Geometry: final body of the model. Coordinates: model frame, mm. Round coordinates to 2 decimals unless told otherwise and drop trailing zeros. Write each loop counter-clockwise with the first axis right and the second up, starting at its lowest first coordinate (ties: lowest second). Pieces come first, ordered by that corner, then holes. Notation, with made-up numbers: M -37.75,23.25 L -10.75,23.25 A30 cw -10.75,62.25 Z; hole C 17,33 d7. An arc over 180 degrees is marked long. Answer as CSV lines item,"result". Start each with the question number.
Q1. Mould query, pull axis Y, two halves, no side actions, for faces 1 (the flat face through (-26.69, -18.86, 8.52)), 2 (the cylindrical face through (30.24, -3.65, -0.14)), 3 (the flat face through (26.69, 18.86, 8.52)). Classes: pulls with the +Y half, pulls with the -Y half, needs draft (parallel to the pull), parting line crosses it, or undercut.
Q2. Ray query, probe 1 along X at (y, z) = (-9, 3.5); probe 2 along Y at (x, z) = (17.5, 9.25); probe 3 along Y at (x, z) = (-29.5, 1.75). Return the intervals inside material, ascending.
Q3. Section query D-D on x = 35. Output: boundary loops of the cut face in (y, z), and give its area (3 significant figures).
Q4. Section query C-C on x = 0. Output: boundary loops of the cut face in (y, z).
Q5. Section query B-B on y = 0. Output: boundary loops of the cut face in (x, z), and give its area (3 significant figures).
Q6. First-contact query: pin 1 (10 mm diameter, centred on x = -28, z = 3, fed in from +Y); pin 2 (10 mm diameter, centred on x = -36, z = -6.5, fed in from -Y); pin 3 (8 mm diameter, centred on y = -21.5, z = 6, fed in from -X). Flat tips, straight axial feed; report the tip coordinate or a pass-through.
Q7. Section query A-A on z = -1.25. Output: boundary loops of the cut face in (x, y).
```python
from build123d import *

# Parameters (mm, degrees)
F0_R     = 6
F0_R_2   = 21
F1_DEPTH = 10
F2_SIZE  = 3


with BuildPart() as f1:
    # F0 (on Top) → F1 (new body)
    with BuildSketch(Plane.XY):
        with BuildLine():
            Line((41.428571, 13.552619), (12.857143, 27.105237))
            ThreePointArc((12.857143, 27.105237), (0, 30), (-12.857143, 27.105237))
            Line((-12.857143, 27.105237), (-41.428571, 13.552619))
            ThreePointArc((-41.428571, 13.552619), (-50, 0), (-41.428571, -13.552619))
            Line((-41.428571, -13.552619), (-12.857143, -27.105237))
            ThreePointArc((-12.857143, -27.105237), (0, -30), (12.857143, -27.105237))
            Line((12.857143, -27.105237), (41.428571, -13.552619))
            ThreePointArc((41.428571, -13.552619), (50, 0), (41.428571, 13.552619))
        make_face()
        with Locations((-35, 0)):
            Circle(F0_R, mode=Mode.SUBTRACT)
        Circle(F0_R_2, mode=Mode.SUBTRACT)
        with Locations((35, 0)):
            Circle(F0_R, mode=Mode.SUBTRACT)
    extrude(amount=F1_DEPTH)

    # F2
    f2_edges = [f1.edges().sort_by_distance(p)[0] for p in [
        (-27.142857, -20.328928, 10),
        (0, -30, 10),
        (27.142857, -20.328928, 10),
    ]]
    chamfer(f2_edges, length=F2_SIZE)

    # F3: F1 across face


with BuildPart() as f1_1:
    add(f1.part)
    add(f1.part.mirror(Plane(origin=(0, 0, 0), x_dir=(1, 0, 0), z_dir=(0, 0, -1))))


solid = f1_1.part
```
Entries:
1,face 1,"pulls with the -Y half"
1,face 2,"undercut"
1,face 3,"pulls with the +Y half"
2,probe 1,"x = -47 to -18.97, 18.97 to 47"
2,probe 2,"y = -22.41 to -11.61, 11.61 to 22.41"
2,probe 3,"y = -19.21 to -2.4, 2.4 to 19.21"
3,outline,"M -16.6,-7 L -13.28,-10 L -6,-10 L -6,10 L -13.28,10 L -16.6,7 Z; M 6,-10 L 13.28,-10 L 16.6,-7 L 16.6,7 L 13.28,10 L 6,10 Z"
3,area,"404 mm^2"
4,outline,"M -30,-7 L -27,-10 L -21,-10 L -21,10 L -27,10 L -30,7 Z; M 21,-10 L 27,-10 L 30,-7 L 30,7 L 27,10 L 21,10 Z"
5,outline,"M -50,-7 L -47,-10 L -41,-10 L -41,10 L -47,10 L -50,7 Z; M -29,-10 L -21,-10 L -21,10 L -29,10 Z; M 21,-10 L 29,-10 L 29,10 L 21,10 Z; M 41,-10 L 47,-10 L 50,-7 L 50,7 L 47,10 L 41,10 Z"
5,area,"662 mm^2"
6,pin 1,"stops at y = 22.29"
6,pin 2,"stops at y = -18.5"
6,pin 3,"stops at x = -33.11"
7,outline,"M -41.43,-13.55 L -12.86,-27.11 A30 ccw 12.86,-27.11 L 41.43,-13.55 A15 ccw 41.43,13.55 L 12.86,27.11 A30 ccw -12.86,27.11 L -41.43,13.55 A15 ccw Z; hole C -35,0 d12; hole C 0,0 d42; hole C 35,0 d12"
